Can you work these out from the model? Positions are in its coordinate system, mm. Face numbers are marked on the shaded views. Coordinates: 2 decimals unless noted, no trailing zeros. Order: outer loops, then holes, each group sorted by start corner. A loop starts at its lowest first (then second) coordinate and runs counter-clockwise, first axis right, second up. Notation, with made-up numbers: (17, -32.5) -> (56, -32.5) arc R26 cw to (56, -12.5) -> close; hole circle Ø10 at (89, 9.5). An arc over 180 degrees is marked (long way). Answer as a JSON object with one key per item and string values. Group by question number.
(1) I want a section at B-B, the plane y = 1. List the corners of the cut face in (x, z) for me, plus the area to 3 significant figures.
(2) I want a section at A-A, the plane x = 20. List the corners of the cut face in (y, z) for me, plus the area to 3 significant figures.
(3) I need wall thicknesses on line 1 (X direction, y = 7.5, z = 6); line 2 (X direction, y = 8.5, z = 4.75); line 3 (Z direction, x = 12, y = 7.6). Which ranges of each line are inside material? Lowest first, please.
(4) If we mould it in two halves opening along Z, with no side actions, what happens to the marked faces 1, 2 and 3? For each: pulls with the +Z half, pulls with the -Z half, needs draft (parallel to the pull), parting line crosses it, or undercut.
(5) For pin 1 (5.5 mm diameter, centred on x = 12, z = 6, fed in from -Y); pin 2 (3.5 mm diameter, centred on x = 4, z = 6, fed in from -Y), each with a flat end and sliding along its axis, tell me the tip position at first contact or that it passes through.
(6) I want a section at D-D, the plane y = 5.5. List the corners of the cut face in (x, z) for me.
(7) I want a section at C-C, the plane z = 6. List the corners of the cut face in (x, y) for me.
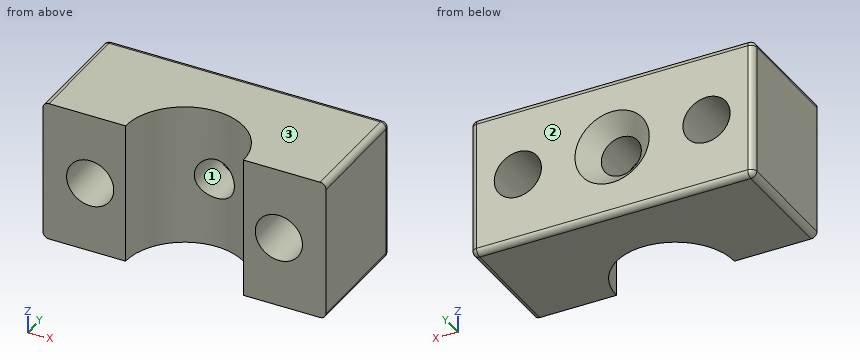
from build123d import *

# Parameters (mm, degrees)
BOSS_EXTRUDE1_DEPTH                             = 12
SKETCH2_R                                       = 2
CUT_EXTRUDE1_DEPTH                              = 29.635642127
CSK_FOR_M3_FLAT_HEAD_MACHINE_SCREW1_D           = 3.4
CSK_FOR_M3_FLAT_HEAD_MACHINE_SCREW1_CSINK_D     = 6.3
CSK_FOR_M3_FLAT_HEAD_MACHINE_SCREW1_CSINK_ANGLE = 90
FILLET1_R                                       = 0.5


with BuildPart() as part:
    # Sketch1 → Boss-Extrude1 (new body)
    with BuildSketch(Plane.XY):
        with BuildLine():
            Line((17, 0), (24, 0))
            Line((24, 0), (24, 10))
            Line((24, 10), (0, 10))
            Line((0, 10), (0, 0))
            Line((0, 0), (7, 0))
            ThreePointArc((7, 0), (12, 5), (17, 0))
        make_face()
    extrude(amount=BOSS_EXTRUDE1_DEPTH)

    # Sketch2 → Cut-Extrude1 (cut, through all)
    with BuildSketch(Plane(origin=(0, 10, 0), x_dir=(1, 0, 0), z_dir=(0, 1, 0))):
        with Locations(Location((4, -6, 0), (0, 0, 270))):
            Circle(SKETCH2_R)
        with Locations(Location((20, -6, 0), (0, 0, 270))):
            Circle(SKETCH2_R)
    extrude(amount=-CUT_EXTRUDE1_DEPTH, mode=Mode.SUBTRACT)

    # CSK for M3 Flat Head Machine Screw1 (through all)
    with Locations(Plane(origin=(0, 10, 0), x_dir=(1, 0, 0), z_dir=(0, 1, 0))):
        with Locations((12, -6)):
            CounterSinkHole(CSK_FOR_M3_FLAT_HEAD_MACHINE_SCREW1_D / 2, CSK_FOR_M3_FLAT_HEAD_MACHINE_SCREW1_CSINK_D / 2, counter_sink_angle=CSK_FOR_M3_FLAT_HEAD_MACHINE_SCREW1_CSINK_ANGLE)

    # Fillet1
    fillet1_edges = [part.edges().sort_by_distance(p)[0] for p in [
        (0, 10, 6),
        (24, 10, 6),
        (24, 5, 12),
        (12, 10, 12),
        (0, 5, 12),
        (12, 10, 0),
        (24, 5, 0),
        (0, 5, 0),
    ]]
    fillet(fillet1_edges, radius=FILLET1_R)


solid = part.part
Computed values:
{
 "1": {"outline": "(0, 0.5) arc R0.5 ccw to (0.5, 0) -> (7.1, 0) -> (7.1, 12) -> (0.5, 12) arc R0.5 ccw to (0, 11.5) -> close; (16.9, 0) -> (23.5, 0) arc R0.5 ccw to (24, 0.5) -> (24, 11.5) arc R0.5 ccw to (23.5, 12) -> (16.9, 12) -> close; hole circle Ø4 at (4, 6); hole circle Ø4 at (20, 6)", "area": "145 mm2"},
 "2": {"outline": "(0, 0) -> (9.5, 0) arc R0.5 ccw to (10, 0.5) -> (10, 4) -> (0, 4) -> close; (0, 8) -> (10, 8) -> (10, 11.5) arc R0.5 ccw to (9.5, 12) -> (0, 12) -> close", "area": "79.9 mm2"},
 "3": {"line 1": "x = 0 to 2, 6 to 10.3, 13.7 to 18, 22 to 24", "line 2": "x = 0 to 2.44, 5.56 to 10.85, 13.15 to 18.44, 21.56 to 24", "line 3": "z = 0 to 4.3, 7.7 to 12"},
 "4": {"face 1": "undercut", "face 2": "needs draft", "face 3": "pulls with the +Z half"},
 "5": {"pin 1": "stops at y = 4.18", "pin 2": "passes through"},
 "6": {"outline": "(0, 0.5) arc R0.5 ccw to (0.5, 0) -> (23.5, 0) arc R0.5 ccw to (24, 0.5) -> (24, 11.5) arc R0.5 ccw to (23.5, 12) -> (0.5, 12) arc R0.5 ccw to (0, 11.5) -> close; hole circle Ø4 at (4, 6); hole circle Ø3.4 at (12, 6); hole circle Ø4 at (20, 6)"},
 "7": {"outline": "(0, 0) -> (2, 0) -> (2, 10) -> (0.5, 10) arc R0.5 ccw to (0, 9.5) -> close; (6, 0) -> (7, 0) arc R5 cw to (10.3, 4.7) -> (10.3, 8.55) -> (8.85, 10) -> (6, 10) -> close; (13.7, 4.7) arc R5 cw to (17, 0) -> (18, 0) -> (18, 10) -> (15.15, 10) -> (13.7, 8.55) -> close; (22, 0) -> (24, 0) -> (24, 9.5) arc R0.5 ccw to (23.5, 10) -> (22, 10) -> close"}
}
